CAD build for the part. Positions are in the model's coordinates, mm. Face numbers are marked on the shaded views. A direction names the side the tool comes from. Give positions to 0.01 mm unless a question says otherwise; leave off trailing zeros. Loops run counter-clockwise (first coordinate to the right, second up) from the corner with the lowest first, then second, coordinate; pieces in that order, holes last. Notation, with made-up numbers: (18, -25) - (25, -25) arc R20 ccw to (25, -14) - close; hole circle Ø9 at (-33, 86.25). An arc over 180 degrees is marked (long way). Return JSON: item names as keys, results as strings.
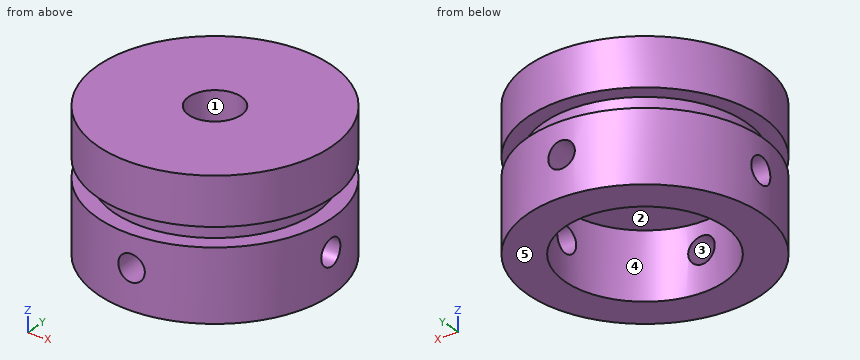
from build123d import *

# Parameters (mm, degrees)
CORTE_EXTRUS_O1_REACH      = 55.104
CORTE_EXTRUS_O1_END_RADIUS = 15
ESBO_O3_R                  = 2.5
PADR_OCIRCULAR1_COUNT      = 4
CORTE_EXTRUS_O2_REACH      = 35.53
ESBO_O5_R                  = 4.95
ESBO_O6_R                  = 22
ESBO_O6_R_2                = 4.95
RESSALTO_EXTRUS_O1_DEPTH   = 6


with BuildPart() as part:
    # Esbo_o1 → Revolu_o1 (revolve)
    with BuildSketch(Plane(origin=(0, 0, 0), x_dir=(1, 0, 0), z_dir=(0, 1, 0)), mode=Mode.PRIVATE) as revolu_o1_sk:
        Polygon((0, 0), (-22, 0), (-22, 3), (-19, 3), (-19, 6.6), (-22, 6.6), (-22, 20), (-15, 20), (-15, 7.5), (0, 7.5), align=None)
    revolve(revolu_o1_sk.sketch.rotate(Axis((0, 0, 0), (0, 0, -1)), 180), axis=Axis((0, 0, 0), (0, 0, -1)))

    # Corte-extrus_o1: up to this cylinder (the profile starts outside it)
    corte_extrus_o1_end = Plane(origin=(0, 0, -12.5), z_dir=(0, 0, 1)) * Cylinder(CORTE_EXTRUS_O1_END_RADIUS, 141.208, mode=Mode.PRIVATE)
    # Esbo_o3 → Corte-extrus_o1 (cut, up to the surface)
    with BuildSketch(Plane.ZY.offset(22), mode=Mode.PRIVATE) as corte_extrus_o1_sk1:
        with Locations((-12.5, 0)):
            Circle(ESBO_O3_R)
    corte_extrus_o1_tool1 = extrude(corte_extrus_o1_sk1.sketch, amount=-CORTE_EXTRUS_O1_REACH, mode=Mode.PRIVATE) - corte_extrus_o1_end
    corte_extrus_o1 = corte_extrus_o1_tool1.solids().sort_by_distance((-22, 0, -12.5))[0]
    add(corte_extrus_o1, mode=Mode.SUBTRACT)

    # Padr_oCircular1: Corte-extrus_o1 ×4 about axis
    padr_ocircular1_axis = Axis((0, 0, -20), (0, 0, 1))
    for i in range(1, PADR_OCIRCULAR1_COUNT):
        add(corte_extrus_o1.rotate(padr_ocircular1_axis, i * 360 / PADR_OCIRCULAR1_COUNT), mode=Mode.SUBTRACT)

    # Esbo_o5 → Corte-extrus_o2 (cut, up to next)
    with BuildSketch(Plane(origin=(0, 0, -7.5), x_dir=(-1, 0, 0), z_dir=(0, 0, -1)), mode=Mode.PRIVATE) as corte_extrus_o2_sk1:
        Circle(ESBO_O5_R)
    corte_extrus_o2_tool1 = extrude(corte_extrus_o2_sk1.sketch, amount=-CORTE_EXTRUS_O2_REACH, mode=Mode.PRIVATE) & part.part
    add(corte_extrus_o2_tool1.solids().sort_by_distance((0, 0, -7.5))[0], mode=Mode.SUBTRACT)

    # Esbo_o6 → Ressalto-extrus_o1 (add)
    with BuildSketch(Plane.XY):
        Circle(ESBO_O6_R)
        with Locations(Location((0, 0, 0), (0, 0, 180))):
            Circle(ESBO_O6_R_2, mode=Mode.SUBTRACT)
    extrude(amount=RESSALTO_EXTRUS_O1_DEPTH)


solid = part.part
1. Drop flat-ended pins along their axis: P1, Ø5, axis at x = 14.5, z = 3.5, coming from the +Y side; P2, Ø4, axis at x = 3, z = -9, coming from the +Y side; P3, Ø5, axis at y = -17, z = -7.5, coming from the +X side. Give the stop position or say it passes through.
Values follow:
{"P1": "stops at y = 18.44", "P2": "stops at y = 21.98", "P3": "stops at x = 16.55"}
2. Which spindle directions (+Z, -Z, +X, -X, +Y, -Y) get a long thin tool onto all of the face, cutting with end or side? Do the marked faces 4 and 5. Say none if no direction does.
Values follow:
{"face 4": "-Z", "face 5": "-Z, +X, -X, +Y, -Y"}
3. Cut at A-A, the plane y = 0. Write the cut outline in (x, z), plus the area to 3 significant figures.
Values follow:
{"outline": "(-22, -20) - (-15, -20) - (-15, -15) - (-22, -15) - close; (-22, -10) - (-15, -10) - (-15, -7.5) - (-4.95, -7.5) - (-4.95, 6) - (-22, 6) - (-22, -3) - (-19, -3) - (-19, -6.6) - (-22, -6.6) - close; (4.95, -7.5) - (15, -7.5) - (15, -10) - (22, -10) - (22, -6.6) - (19, -6.6) - (19, -3) - (22, -3) - (22, 6) - (4.95, 6) - close; (15, -20) - (22, -20) - (22, -15) - (15, -15) - close", "area": "544 mm²"}
4. Cut at C-C, the plane z = -10.75. Write the cut outline in (x, y), plus the area to 3 significant figures.
Values follow:
{"outline": "(-21.93, -1.79) arc R22 ccw to (-1.79, -21.93) - (-1.79, -14.89) arc R15 cw to (-14.89, -1.79) - close; (-21.93, 1.79) - (-14.89, 1.79) arc R15 cw to (-1.79, 14.89) - (-1.79, 21.93) arc R22 ccw to start; (1.79, -21.93) arc R22 ccw to (21.93, -1.79) - (14.89, -1.79) arc R15 cw to (1.79, -14.89) - close; (1.79, 14.89) arc R15 cw to (14.89, 1.79) - (21.93, 1.79) arc R22 ccw to (1.79, 21.93) - close", "area": "714 mm²"}
5. Pull direction Z, two halves, no side cores. Call the marked faces 1, 2 and 3: +Z half, -Z half, draft (parallel to the pull), parting line (faces both ways), or undercut.
Values follow:
{"face 1": "draft", "face 2": "-Z half", "face 3": "undercut"}
6. Drill centre lines: probe 1 along Z at (x, y) = (0, -16); probe 2 along X at (y, z) = (0, 3). Where is each one in solid material? Low to high.
Values follow:
{"probe 1": "z = -20 to -15, -10 to 6", "probe 2": "x = -22 to -4.95, 4.95 to 22"}
7. Cut at D-D, the plane y = -17. Write the cut outline in (x, z), plus the area to 3 significant figures.
Values follow:
{"outline": "(-13.96, -20) - (13.96, -20) - (13.96, -6.6) - (8.49, -6.6) - (8.49, -3) - (13.96, -3) - (13.96, 6) - (-13.96, 6) - (-13.96, -3) - (-8.49, -3) - (-8.49, -6.6) - (-13.96, -6.6) - close; hole circle Ø5 at (0, -12.5)", "area": "667 mm²"}
